```python
from build123d import *

# Parameters (mm, degrees)
SKETCH1_W           = 550
SKETCH1_H           = 350
SKETCH1_W_2         = 432
SKETCH1_H_2         = 158
BASE_FLANGE1_DEPTH  = 4
SKETCH4_W           = 399
SKETCH4_H           = 190
CUT_EXTRUDE1_DEPTH  = 343.669301222
SKETCH5_R           = 2.25
CUT_EXTRUDE2_DEPTH  = 343.669301222
SKETCH6_R           = 1.75
CUT_EXTRUDE3_DEPTH  = 343.669301222
SKETCH8_R           = 2.25
CUT_EXTRUDE5_DEPTH  = 343.669301222
SKETCH10_R          = 2.25
CUT_EXTRUDE7_DEPTH  = 343.669301222
SKETCH11_W          = 7
SKETCH11_H          = 39
TAB1_DEPTH          = 4
SKETCH12_R          = 1.75
CUT_EXTRUDE8_DEPTH  = 343.669301222
CUT_EXTRUDE9_DEPTH  = 343.669301222
SKETCH14_R          = 2.25
CUT_EXTRUDE10_DEPTH = 343.669301222


# Sheet-metal steps are written as plain solids
with BuildPart() as part:
    # Sketch1 → Base-Flange1 (new body)
    with BuildSketch(Plane(origin=(0, 0, 0), x_dir=(1, 0, 0), z_dir=(0, 1, 0))):
        with Locations((-15, 7.5)):
            Rectangle(SKETCH1_W, SKETCH1_H)
        Rectangle(SKETCH1_W_2, SKETCH1_H_2, mode=Mode.SUBTRACT)
    extrude(amount=-BASE_FLANGE1_DEPTH)

    # Sketch4 → Cut-Extrude1 (cut, through all)
    with BuildSketch(Plane(origin=(0, 0, 0), x_dir=(1, 0, 0), z_dir=(0, 1, 0))):
        Rectangle(SKETCH4_W, SKETCH4_H)
    extrude(amount=-CUT_EXTRUDE1_DEPTH, mode=Mode.SUBTRACT)

    # Sketch5 → Cut-Extrude2 (cut, through all)
    with BuildSketch(Plane.XZ.offset(4)):
        with Locations(Location((-254, 71, 0), (0, 0, 270))):
            Circle(SKETCH5_R)
        with Locations(Location((-234, 71, 0), (0, 0, 270))):
            Circle(SKETCH5_R)
        with Locations(Location((-234, -71, 0), (0, 0, 90))):
            Circle(SKETCH5_R)
        with Locations(Location((-254, -71, 0), (0, 0, 90))):
            Circle(SKETCH5_R)
        with Locations(Location((224, 75, 0), (0, 0, 270))):
            Circle(SKETCH5_R)
        with Locations(Location((244, 75, 0), (0, 0, 270))):
            Circle(SKETCH5_R)
        with Locations(Location((224, -75, 0), (0, 0, 90))):
            Circle(SKETCH5_R)
        with Locations(Location((244, -75, 0), (0, 0, 90))):
            Circle(SKETCH5_R)
    extrude(amount=-CUT_EXTRUDE2_DEPTH, mode=Mode.SUBTRACT)

    # Sketch6 → Cut-Extrude3 (cut, through all)
    with BuildSketch(Plane(origin=(0, 0, 0), x_dir=(1, 0, 0), z_dir=(0, 1, 0))):
        with Locations(Location((-225.5, 102, 0), (0, 0, 270))):
            Circle(SKETCH6_R)
        with Locations(Location((-225.5, 121, 0), (0, 0, 270))):
            Circle(SKETCH6_R)
        with Locations(Location((225.5, 102, 0), (0, 0, 90))):
            Circle(SKETCH6_R)
        with Locations(Location((225.5, 121, 0), (0, 0, 90))):
            Circle(SKETCH6_R)
    extrude(amount=-CUT_EXTRUDE3_DEPTH, mode=Mode.SUBTRACT)

    # Sketch8 → Cut-Extrude5 (cut, through all)
    with BuildSketch(Plane(origin=(0, 0, 0), x_dir=(1, 0, 0), z_dir=(0, 1, 0))):
        with Locations(Location((-232, 146.5, 0), (0, 0, 270))):
            Circle(SKETCH8_R)
        with Locations(Location((-232, 166.5, 0), (0, 0, 270))):
            Circle(SKETCH8_R)
        with Locations(Location((-232, -151.5, 0), (0, 0, 270))):
            Circle(SKETCH8_R)
        with Locations(Location((-232, -131.5, 0), (0, 0, 270))):
            Circle(SKETCH8_R)
        with Locations(Location((236, 146.5, 0), (0, 0, 270))):
            Circle(SKETCH8_R)
        with Locations(Location((236, 166.5, 0), (0, 0, 270))):
            Circle(SKETCH8_R)
        with Locations(Location((236, -151.5, 0), (0, 0, 270))):
            Circle(SKETCH8_R)
        with Locations(Location((236, -131.5, 0), (0, 0, 270))):
            Circle(SKETCH8_R)
    extrude(amount=-CUT_EXTRUDE5_DEPTH, mode=Mode.SUBTRACT)

    # Sketch10 → Cut-Extrude7 (cut, through all)
    with BuildSketch(Plane(origin=(0, 0, 0), x_dir=(1, 0, 0), z_dir=(0, 1, 0))):
        with Locations(Location((-284, -147.5, 0), (0, 0, 270))):
            Circle(SKETCH10_R)
        with BuildLine():
            Line((-154, -145.25), (-144, -145.25))
            ThreePointArc((-144, -145.25), (-141.75, -147.5), (-144, -149.75))
            Line((-144, -149.75), (-154, -149.75))
            ThreePointArc((-154, -149.75), (-156.25, -147.5), (-154, -145.25))
        make_face()
    extrude(amount=-CUT_EXTRUDE7_DEPTH, mode=Mode.SUBTRACT)

    # Sketch11 → Tab1 (add)
    with BuildSketch(Plane(origin=(0, 0, 0), x_dir=(1, 0, 0), z_dir=(0, 1, 0))):
        with Locations((-212.5, 0)):
            Rectangle(SKETCH11_W, SKETCH11_H)
        with Locations((212.5, 0)):
            Rectangle(SKETCH11_W, SKETCH11_H)
    extrude(amount=-TAB1_DEPTH)

    # Sketch12 → Cut-Extrude8 (cut, through all)
    with BuildSketch(Plane(origin=(0, 0, 0), x_dir=(1, 0, 0), z_dir=(0, 1, 0))):
        with Locations(Location((-214, 0, 0), (0, 0, 270))):
            Circle(SKETCH12_R)
        with Locations(Location((214, 0, 0), (0, 0, 270))):
            Circle(SKETCH12_R)
    extrude(amount=-CUT_EXTRUDE8_DEPTH, mode=Mode.SUBTRACT)

    # Sketch13 → Cut-Extrude9 (cut, through all)
    with BuildSketch(Plane(origin=(0, 0, 0), x_dir=(1, 0, 0), z_dir=(0, 1, 0))):
        with BuildLine():
            Line((-221, -27.5), (169.756928825, -27.5))
            ThreePointArc((169.756928825, -27.5), (179.756928825, -37.5), (169.756928825, -47.5))
            Line((169.756928825, -47.5), (-221, -47.5))
            ThreePointArc((-221, -47.5), (-231, -37.5), (-221, -27.5))
        make_face()
        with BuildLine():
            Line((-221, 27.5), (169.756928825, 27.5))
            ThreePointArc((169.756928825, 27.5), (179.756928825, 37.5), (169.756928825, 47.5))
            Line((169.756928825, 47.5), (-221, 47.5))
            ThreePointArc((-221, 47.5), (-231, 37.5), (-221, 27.5))
        make_face()
    extrude(amount=-CUT_EXTRUDE9_DEPTH, mode=Mode.SUBTRACT)

    # Sketch14 → Cut-Extrude10 (cut, through all)
    with BuildSketch(Plane(origin=(0, 0, 0), x_dir=(1, 0, 0), z_dir=(0, 1, 0))):
        with Locations(Location((-281.5, 37.5, 0), (0, 0, 270))):
            Circle(SKETCH14_R)
        with Locations(Location((-256.5, 37.5, 0), (0, 0, 270))):
            Circle(SKETCH14_R)
        with Locations(Location((-281.5, -37.5, 0), (0, 0, 270))):
            Circle(SKETCH14_R)
        with Locations(Location((-256.5, -37.5, 0), (0, 0, 270))):
            Circle(SKETCH14_R)
    extrude(amount=-CUT_EXTRUDE10_DEPTH, mode=Mode.SUBTRACT)


solid = part.part
```
Could you check a few things on this model? Use its own coordinates, in mm. Round coordinates to 2 decimals unless told otherwise and drop trailing zeros. Loops run counter-clockwise (first coordinate to the right, second up) from the corner with the lowest first, then second, coordinate; pieces in that order, holes last. Notation, with made-up numbers: (-24, 78) - (19, 78) arc R36 ccw to (19, 115) - close; hole circle Ø4 at (-20.5, 80). An arc over 180 degrees is marked (long way). Answer in a Markdown table with one row per item. Add a question column.
(1) If we section it at C-C (y = -1.65): State how many separate pieces and enclosed holes the cut face has, plus the area to 3 significant figures.
(2) I need wall thicknesses on line 1 along X through (y, z) = (-0.95, -166.5); line 2 along Z through (x, y) = (-281.5, -1.25); line 3 along Z through (x, y) = (214, -1.2). Which ranges of each line are inside material? Lowest first, please.
(3) I'm going to push a flat-ended pin straight in: pin 1 (3 mm diameter, centred on x = -214, z = 0, fed in from -Y). Where does the tip first touch, or does it pass through?
(4) If we section it at A-A (x = 106): Please give me the cut outline in (y, z), plus the area to 3 significant figures.
(5) If we section it at B-B (z = 57.5): Please give me the cut outline in (x, y), plus the area to 3 significant figures.
(6) If we mould it in two halves opening along X, with no side actions, what happens to faces 1 (the face through (-19, -4, -127)), 2 (the face through (-231, -2, -37.7)), 3 (the face through (-231, -2, 37.7))? For each: pulls with the +X half, pulls with the -X half, needs draft (parallel to the pull), parting line crosses it, or undercut.
Model answer:
| question | item | result |
|---|---|---|
| 1 | separate pieces | 1 |
| 1 | enclosed holes | 29 |
| 1 | area | 111,000 mm² |
| 2 | line 1 | x = -290 to -234.25, -229.75 to 233.75, 238.25 to 260 |
| 2 | line 2 | z = -182.5 to -39.75, -35.25 to 35.25, 39.75 to 167.5 |
| 2 | line 3 | z = -182.5 to -79, -19.5 to -1.75, 1.75 to 19.5, 79 to 167.5 |
| 3 | pin 1 | passes through |
| 4 | outline | (-4, -182.5) - (0, -182.5) - (0, -95) - (-4, -95) - close; (-4, 95) - (0, 95) - (0, 167.5) - (-4, 167.5) - close |
| 4 | area | 640 mm² |
| 5 | outline | (-290, -4) - (-216, -4) - (-216, 0) - (-290, 0) - close; (216, -4) - (260, -4) - (260, 0) - (216, 0) - close |
| 5 | area | 472 mm² |
| 6 | face 1 | needs draft |
| 6 | face 2 | undercut |
| 6 | face 3 | undercut |
